```python
from build123d import *

# Parameters (mm, degrees)
F1_DEPTH = 10.75
F2_R     = 4
F3_DEPTH = 16.75
F5_DEPTH = 25.75


with BuildPart() as f1:
    # F0 (on Top) → F1 (new body)
    with BuildSketch(Plane.XY):
        with BuildLine():
            Line((0, 0), (7.2, 0))
            ThreePointArc((7.2, 0), (7.1656564529, 0.7024013095), (7.0629534446, 1.3981017988))
            ThreePointArc((7.0629534446, 1.3981017988), (6.2353829072, 3.6), (4.7422683972, 5.4176462093))
            ThreePointArc((4.7422683972, 5.4176462093), (4.1911256041, 5.8544398682), (3.6, 6.2353829072))
            Line((3.6, 6.2353829072), (0, 0))
        make_face()
        with BuildLine():
            Line((8.025, 0), (7.2, 0))
            ThreePointArc((7.2, 0), (7.1656564529, -0.7024013095), (7.0629534446, -1.3981017988))
            Line((7.0629534446, -1.3981017988), (9.1264666645, -0.845185098))
            ThreePointArc((9.1264666645, -0.845185098), (8.3673337496, -0.6941841728), (8.025, 0))
        make_face()
        with BuildLine():
            ThreePointArc((7.0629534446, -1.3981017988), (7.1656564529, -0.7024013095), (7.2, 0))
            Line((7.2, 0), (0, 0))
            Line((0, 0), (-6.5254160667, -3.0428514845))
            ThreePointArc((-6.5254160667, -3.0428514845), (-6.197442622, -3.6649290508), (-5.8103463543, -4.2520436549))
            ThreePointArc((-5.8103463543, -4.2520436549), (1.5583652204, -7.0293312513), (7.0629534446, -1.3981017988))
        make_face()
        with BuildLine():
            ThreePointArc((7.0629534446, 1.3981017988), (7.1656564529, 0.7024013095), (7.2, 0))
            Line((7.2, 0), (8.025, 0))
            ThreePointArc((8.025, 0), (8.3673337496, 0.6941841728), (9.1264666645, 0.845185098))
            Line((9.1264666645, 0.845185098), (7.0629534446, 1.3981017988))
        make_face()
        with BuildLine():
            Line((-4.1297503417, 5.8978947189), (0, 0))
            Line((0, 0), (3.6, 6.2353829072))
            ThreePointArc((3.6, 6.2353829072), (2.9745308488, 6.5568411777), (2.3206850474, 6.8157480082))
            ThreePointArc((2.3206850474, 6.8157480082), (-0.314059589, 7.1931471954), (-2.9058857202, 6.5875510003))
            ThreePointArc((-2.9058857202, 6.5875510003), (-3.5346782238, 6.272642972), (-4.1297503417, 5.8978947189))
        make_face()
        with BuildLine():
            Line((-6.5254160667, -3.0428514845), (0, 0))
            Line((0, 0), (-4.1297503417, 5.8978947189))
            ThreePointArc((-4.1297503417, 5.8978947189), (-4.6854251609, 5.466881292), (-5.1964016135, 4.9837145054))
            ThreePointArc((-5.1964016135, 4.9837145054), (-6.9546659493, 1.8634971247), (-6.9920730582, -1.7178225601))
            ThreePointArc((-6.9920730582, -1.7178225601), (-6.7911378629, -2.3917454979), (-6.5254160667, -3.0428514845))
        make_face()
        with BuildLine():
            ThreePointArc((9.1264666645, 0.845185098), (8.3673337496, 0.6941841728), (8.025, 0))
            Line((8.025, 0), (8.9, 0))
            Line((8.9, 0), (9.1264666645, 0.845185098))
        make_face()
        with BuildLine():
            Line((8.9, 0), (8.025, 0))
            ThreePointArc((8.025, 0), (8.3673337496, -0.6941841728), (9.1264666645, -0.845185098))
            Line((9.1264666645, -0.845185098), (8.9, 0))
        make_face()
        with BuildLine():
            ThreePointArc((3.6, 6.2353829072), (4.1911256041, 5.8544398682), (4.7422683972, 5.4176462093))
            Line((4.7422683972, 5.4176462093), (5.295185098, 7.4811594292))
            ThreePointArc((5.295185098, 7.4811594292), (4.7848480033, 6.8992315027), (4.0125, 6.9498538654))
            Line((4.0125, 6.9498538654), (3.6, 6.2353829072))
        make_face()
        with BuildLine():
            ThreePointArc((9.775, 0), (9.5941841728, 0.5326662504), (9.1264666645, 0.845185098))
            Line((9.1264666645, 0.845185098), (8.9, 0))
            Line((8.9, 0), (9.1264666645, -0.845185098))
            ThreePointArc((9.1264666645, -0.845185098), (9.5941841728, -0.5326662504), (9.775, 0))
        make_face()
        with BuildLine():
            Line((-7.9141971492, -4.6230093134), (-5.8103463543, -4.2520436549))
            ThreePointArc((-5.8103463543, -4.2520436549), (-6.197442622, -3.6649290508), (-6.5254160667, -3.0428514845))
            Line((-6.5254160667, -3.0428514845), (-7.273119991, -3.3915115505))
            ThreePointArc((-7.273119991, -3.3915115505), (-7.2118802984, -3.5719178673), (-7.1911393046, -3.7613025295))
            ThreePointArc((-7.1911393046, -3.7613025295), (-7.3958504169, -4.323741688), (-7.9141971492, -4.6230093134))
        make_face()
        with BuildLine():
            Line((-7.273119991, -3.3915115505), (-6.5254160667, -3.0428514845))
            ThreePointArc((-6.5254160667, -3.0428514845), (-6.7911378629, -2.3917454979), (-6.9920730582, -1.7178225601))
            Line((-6.9920730582, -1.7178225601), (-8.6285784631, -3.0910136418))
            ThreePointArc((-8.6285784631, -3.0910136418), (-7.8767546424, -2.9070435233), (-7.273119991, -3.3915115505))
        make_face()
        with BuildLine():
            ThreePointArc((2.3206850474, 6.8157480082), (2.9745308488, 6.5568411777), (3.6, 6.2353829072))
            Line((3.6, 6.2353829072), (4.0125, 6.9498538654))
            ThreePointArc((4.0125, 6.9498538654), (3.5824857463, 7.5934156755), (3.8312815665, 8.3263445272))
            Line((3.8312815665, 8.3263445272), (2.3206850474, 6.8157480082))
        make_face()
        with BuildLine():
            Line((-4.6029509017, 6.5736951554), (-4.1297503417, 5.8978947189))
            ThreePointArc((-4.1297503417, 5.8978947189), (-3.5346782238, 6.272642972), (-2.9058857202, 6.5875510003))
            Line((-2.9058857202, 6.5875510003), (-4.542391125, 7.9607420819))
            ThreePointArc((-4.542391125, 7.9607420819), (-4.3118109699, 7.6602441732), (-4.2298302835, 7.2904531942))
            ThreePointArc((-4.2298302835, 7.2904531942), (-4.3286958045, 6.8864231576), (-4.6029509017, 6.5736951554))
        make_face()
        with BuildLine():
            ThreePointArc((-5.1964016135, 4.9837145054), (-4.6854251609, 5.466881292), (-4.1297503417, 5.8978947189))
            Line((-4.1297503417, 5.8978947189), (-4.6029509017, 6.5736951554))
            ThreePointArc((-4.6029509017, 6.5736951554), (-5.3679478581, 6.4559508623), (-5.9270613267, 6.9911855688))
            Line((-5.9270613267, 6.9911855688), (-5.1964016135, 4.9837145054))
        make_face()
        with BuildLine():
            Line((4.45, 7.7076260937), (5.295185098, 7.4811594292))
            ThreePointArc((5.295185098, 7.4811594292), (5.3175142537, 7.5934156755), (5.325, 7.7076260937))
            ThreePointArc((5.325, 7.7076260937), (4.7848480033, 8.5160206846), (3.8312815665, 8.3263445272))
            Line((3.8312815665, 8.3263445272), (4.45, 7.7076260937))
        make_face()
        with BuildLine():
            ThreePointArc((4.0125, 6.9498538654), (4.7848480033, 6.8992315027), (5.295185098, 7.4811594292))
            Line((5.295185098, 7.4811594292), (4.45, 7.7076260937))
            Line((4.45, 7.7076260937), (4.0125, 6.9498538654))
        make_face()
        with BuildLine():
            ThreePointArc((-8.6285784631, -3.0910136418), (-8.8591586183, -4.1310935085), (-7.9141971492, -4.6230093134))
            ThreePointArc((-7.9141971492, -4.6230093134), (-7.3958504169, -4.323741688), (-7.1911393046, -3.7613025295))
            ThreePointArc((-7.1911393046, -3.7613025295), (-7.2118802984, -3.5719178673), (-7.273119991, -3.3915115505))
            ThreePointArc((-7.273119991, -3.3915115505), (-7.8767546424, -2.9070435233), (-8.6285784631, -3.0910136418))
        make_face()
        with BuildLine():
            ThreePointArc((3.8312815665, 8.3263445272), (3.5824857463, 7.5934156755), (4.0125, 6.9498538654))
            Line((4.0125, 6.9498538654), (4.45, 7.7076260937))
            Line((4.45, 7.7076260937), (3.8312815665, 8.3263445272))
        make_face()
        with BuildLine():
            ThreePointArc((-5.9270613267, 6.9911855688), (-5.3679478581, 6.4559508623), (-4.6029509017, 6.5736951554))
            ThreePointArc((-4.6029509017, 6.5736951554), (-4.3286958045, 6.8864231576), (-4.2298302835, 7.2904531942))
            ThreePointArc((-4.2298302835, 7.2904531942), (-4.3118109699, 7.6602441732), (-4.542391125, 7.9607420819))
            ThreePointArc((-4.542391125, 7.9607420819), (-5.6067096653, 8.0072112329), (-5.9270613267, 6.9911855688))
        make_face()
    extrude(amount=F1_DEPTH)

    # F2 (on face) → F3 (join)
    with BuildSketch(Plane.XY.offset(10.75)):
        Circle(F2_R)
    extrude(amount=-F3_DEPTH)

    # F4 (on face) → F5 (join)
    with BuildSketch(Plane(origin=(0, 0, 0), x_dir=(1, 0, 0), z_dir=(0, 0, -1))):
        with BuildLine():
            Line((1.5320888862, 1.2855752194), (-0.6945927107, 3.939231012))
            ThreePointArc((-0.6945927107, 3.939231012), (-3.0641777725, -2.5711504387), (3.7587704831, -1.3680805733))
            Line((3.7587704831, -1.3680805733), (1.5320888862, 1.2855752194))
        make_face()
    extrude(amount=-F5_DEPTH)


solid = f1.part
```
Check sheet for the modelled part. Datum: model origin and axes. Units: mm. A direction names the side the tool comes from. Give positions to 0.01 mm unless a question says otherwise; leave off trailing zeros. Write each loop counter-clockwise with the first axis right and the second up, starting at its lowest first coordinate (ties: lowest second). Pieces come first, ordered by that corner, then holes. Notation, with made-up numbers: (39.25, 58) - (60.25, 58) arc R25 ccw to (60.25, 92) - close; hole circle Ø6 at (-18.75, 7.5). An arc over 180 degrees is marked (long way). Answer as a JSON object with one key per item and string values. Group by question number.
1) Sectioned sample at B-B (y = 3). Record the cut outline in (x, z).
2) Sectioned sample at C-C (x = 0). Record the cut outline in (y, z), then the cut area to 3 significant figures.
3) Depth check by flat-ended pin: P1, Ø8, axis at x = -5, z = 15.5, coming from the +Y side; P2, Ø3, axis at y = 4.5, z = 8, coming from the -X side; P3, Ø3, axis at y = 2.5, z = 14.5, coming from the +X side. Enter the tip coordinate at first touch or a pass-through.
4) Access from +Z, -Z, +X, -X, +Y, -Y to the whole of each face (thin tool, end or side, straight path). Record for faces 1 (the face through (-0.867, -3.905, -2.958)), 2 (the face through (-6.88, -4.44, 5.3)), 3 (the face through (3.087, 7.582, 5.3)).
5) Thickness scan on probe 1 along Z at (x, y) = (-4.5, 6); probe 2 along Z at (x, y) = (1.5, -2); probe 3 along X at (y, z) = (0.25, 20). Record the ranges inside material, lowest first. Write a range as from..to.
6) Sectioned sample at A-A (z = 3). Record the cut outline in (x, y) (3 decimals).
7) Release check for a two-part mould opening along Y. For faces 4 (the face through (-3.14, 2.48, 18.14)), 5 (the face through (2, -1, 10.75)), 6 (the face through (5.015, 6.435, 5.3)), 7 (the face through (-6.94, 1.91, 5.3)) record: pulls with the +Y half, pulls with the -Y half, needs draft (parallel to the pull), parting line crosses it, or undercut.
8) Sectioned sample at D-D (z = 19). Record the cut outline in (x, y).
Geometry results:
{
 "1": {"outline": "(-6.55, 0) - (-2.65, 0) - (-2.65, -6) - (2.65, -6) - (2.65, 0) - (6.55, 0) - (6.55, 10.75) - (2.65, 10.75) - (2.65, 25.75) - (-2.65, 25.75) - (-2.65, 10.75) - (-6.55, 10.75) - close"},
 "2": {"outline": "(-7.2, 0) - (-4, 0) - (-4, -6) - (4, -6) - (4, 0) - (7.2, 0) - (7.2, 10.75) - (4, 10.75) - (4, 25.75) - (-3.11, 25.75) - (-3.11, 10.75) - (-7.2, 10.75) - close", "area": "309 mm^2"},
 "3": {"P1": "stops at y = 3.87", "P2": "stops at x = -6.55", "P3": "stops at x = 3.76"},
 "4": {"face 1": "-Z", "face 2": "+Z, -Z, -Y", "face 3": "+Z, -Z, +Y"},
 "5": {"probe 1": "z = 0..10.75", "probe 2": "z = -6..10.75", "probe 3": "x = -3.99..2.82"},
 "6": {"outline": "(-8.629, -3.091) arc R0.875 ccw to (-7.914, -4.623) - (-5.81, -4.252) arc R7.2 ccw to (7.063, -1.398) - (9.126, -0.845) arc R0.875 ccw to (9.126, 0.845) - (7.063, 1.398) arc R7.2 ccw to (4.742, 5.418) - (5.295, 7.481) arc R0.875 ccw to (3.831, 8.326) - (2.321, 6.816) arc R7.2 ccw to (-2.906, 6.588) - (-4.542, 7.961) arc R0.875 ccw to (-5.927, 6.991) - (-5.196, 4.984) arc R7.2 ccw to (-6.992, -1.718) - close"},
 "7": {"face 4": "parting line crosses it", "face 5": "needs draft", "face 6": "undercut", "face 7": "undercut"},
 "8": {"outline": "(-0.69, -3.94) - (3.76, 1.37) arc R4 ccw (long way) to start"}
}
